```python
from build123d import *
from build123d.topology import SkipClean

# Parameters (mm, degrees)
SKETCH1_W           = 254.5
SKETCH1_H           = 20
BOSS_EXTRUDE1_DEPTH = 1.5
CUT_REVOLVE1_ANGLE  = 360


with BuildPart() as part:
    # Sketch1 → Boss-Extrude1 (new body, symmetric)
    with BuildSketch(Plane(origin=(0, 0, 0), x_dir=(0, 0, -1), z_dir=(1, 0, 0))):
        with Locations((447.25, 86)):
            Rectangle(SKETCH1_W, SKETCH1_H)
    extrude(amount=BOSS_EXTRUDE1_DEPTH, both=True)

    # Sketch2 → Cut-Revolve1 (revolve, symmetric, cut)
    with SkipClean():  # keep this step's faces unmerged: merging them makes the solid invalid here
        with BuildSketch(Plane(origin=(0, 0, 0), x_dir=(0, 0, -1), z_dir=(1, 0, 0))) as cut_revolve1_sk:
            Polygon((320, 83.6), (331, 83.6), (331, 78.6), (334, 78.6), (334, 83.6), (544, 83.6), (544, 78.6), (547, 78.6), (547, 83.6), (574.5, 83.6), (574.5, 65.235756371), (320, 65.235756371), align=None)
        revolve(axis=Axis((0, 0, 0), (0, 0, -1)), revolution_arc=CUT_REVOLVE1_ANGLE / 2, mode=Mode.SUBTRACT)
        revolve(cut_revolve1_sk.sketch, axis=Axis((0, 0, 0), (0, 0, 1)), revolution_arc=CUT_REVOLVE1_ANGLE / 2, mode=Mode.SUBTRACT)


solid = part.part
```
CAD build for the part. Positions are in the model's coordinates, mm. Give positions to 0.01 mm unless a question says otherwise; leave off trailing zeros. Write each loop counter-clockwise with the first axis right and the second up, starting at its lowest first coordinate (ties: lowest second). Pieces come first, ordered by that corner, then holes. Notation, with made-up numbers: M 25.25,32.5 L 59.25,32.5 A27 ccw 59.25,62.5 Z; hole C 48.25,34 d7. An arc over 180 degrees is marked long. Return JSON: item names as keys, results as strings. Group by question number.
(1) Band-saw the part on C-C (z = -419). Give the cut face in (x, y), and give its area (3 significant figures).
(2) Flat gauge pins, fed straight in: pin 1 Ø1.5 at (x, y) = (0.5, 81.5) entering from -Z; pin 2 Ø0.9 at (x, y) = (0, 82) entering from +Z. Where does each tip first touch, or does it go through?
(3) Drill centre lines: L1, parallel to Z at x = -0.25, y = 82.5; L2, parallel to Y at x = 0.6, z = -557. Where is each one in solid material? Low to high. Write a range as [from, to].
(4) Band-saw the part on B-B (x = -0.6). Give the cut face in (y, z).
(5) Band-saw the part on A-A (y = 81.25). Give the cut face in (x, z), and give its area (3 significant figures).
Entries:
{
 "1": {"outline": "M -1.5,83.59 A83.6 cw 1.5,83.59 L 1.5,96 L -1.5,96 Z", "area": "37.2 mm^2"},
 "2": {"pin 1": "stops at z = -547", "pin 2": "stops at z = -331"},
 "3": {"L1": "z = [-547, -544], [-334, -331]", "L2": "y = [83.6, 96]"},
 "4": {"outline": "M 78.6,-547 L 83.6,-547 L 83.6,-574.5 L 96,-574.5 L 96,-320 L 83.6,-320 L 83.6,-331 L 78.6,-331 L 78.6,-334 L 83.6,-334 L 83.6,-544 L 78.6,-544 Z"},
 "5": {"outline": "M -1.5,-547 L 1.5,-547 L 1.5,-544 L -1.5,-544 Z; M -1.5,-334 L 1.5,-334 L 1.5,-331 L -1.5,-331 Z", "area": "18.0 mm^2"}
}
